from build123d import *

# Parameters (mm, degrees)
SKETCH1_W                   = 25.4
SKETCH1_H                   = 25.4
SKETCH1_W_2                 = 15.875
SKETCH1_H_2                 = 15.875
BOSS_EXTRUDE1_DEPTH         = 298
FILLET1_R                   = 1.5
F_1_4_0_25_DIAMETER_HOLE1_D = 6.35
SKETCH4_R                   = 2.2
SKETCH4_R_2                 = 2.75
CUT_EXTRUDE1_DEPTH          = 26.4


with BuildPart() as part:
    # Sketch1 → Boss-Extrude1 (new body, symmetric)
    with BuildSketch(Plane(origin=(0, 0, 0), x_dir=(1, 0, 0), z_dir=(0, 1, 0))):
        Rectangle(SKETCH1_W, SKETCH1_H)
        Rectangle(SKETCH1_W_2, SKETCH1_H_2, mode=Mode.SUBTRACT)
    extrude(amount=BOSS_EXTRUDE1_DEPTH, both=True)

    # Fillet1
    fillet1_edges = [part.edges().sort_by_distance(p)[0] for p in [
        (12.7, 0, 12.7),
        (-12.7, 0, 12.7),
        (-12.7, 0, -12.7),
        (12.7, 0, -12.7),
    ]]
    fillet(fillet1_edges, radius=FILLET1_R)

    # 1/4 (0.25) Diameter Hole1 (through all)
    with Locations(Plane(origin=(0.011805537, 289.825, -12.7), x_dir=(-1, 0, 0), z_dir=(0, 0, -1))):
        with Locations((0, 0), (0, -19), (0, -38)):
            f_1_4_0_25_diameter_hole1 = Hole(F_1_4_0_25_DIAMETER_HOLE1_D / 2)

    # Mirror1: 1/4 (0.25) Diameter Hole1 across plane
    add(f_1_4_0_25_diameter_hole1.mirror(Plane.ZX), mode=Mode.SUBTRACT)

    # Sketch4 → Cut-Extrude1 (cut, through all)
    with BuildSketch(Plane.ZY.offset(12.7)):
        with Locations((0, 134.3)):
            Circle(SKETCH4_R)
        with Locations((0, -134.3)):
            Circle(SKETCH4_R)
        with Locations((0, 238.65)):
            Circle(SKETCH4_R_2)
        with Locations((0, 226.9)):
            Circle(SKETCH4_R_2)
        with Locations((0, 215.15)):
            Circle(SKETCH4_R_2)
        with Locations((0, -215.15)):
            Circle(SKETCH4_R_2)
        with Locations((0, -226.9)):
            Circle(SKETCH4_R_2)
        with Locations((0, -238.65)):
            Circle(SKETCH4_R_2)
        with Locations((0, 190)):
            Circle(SKETCH4_R_2)
        with Locations((0, -190)):
            Circle(SKETCH4_R_2)
    extrude(amount=-CUT_EXTRUDE1_DEPTH, mode=Mode.SUBTRACT)


solid = part.part
The model under review builds one solid part; all positions refer to its coordinate system, in mm. A direction names the side the tool comes from. Coordinates: 2 decimals unless noted, no trailing zeros. Write each loop counter-clockwise with the first axis right and the second up, starting at its lowest first coordinate (ties: lowest second). Pieces come first, ordered by that corner, then holes. Notation, with made-up numbers: (-27.5, 43.25) - (10.5, 43.25) arc R28 cw to (10.5, 72.25) - close; hole circle Ø6 at (1.5, 71.5). An arc over 180 degrees is marked (long way). Answer as a JSON object with one key per item and string values. Group by question number.
1. Mouldability with a two-part tool opening along Z and no side actions: class faces 1 (the face through (-7.938, 4, 0)), 2 (the face through (8.3, 298, -0.2)), 3 (the face through (0, 4, 12.7)) as pulls with the +Z half, pulls with the -Z half, needs draft (parallel to the pull), parting line crosses it, or undercut.
2. Add section A-A (y = 119.5). Give the boundary of the cut face in (x, z).
3. To check wall thickness, follow probe 1 along Z at (x, y) = (5.5, 87.5); probe 2 along Z at (x, y) = (-9.6, -215.15). State the ranges of each line that lie inside material, in increasing order.
4. Machinability: for faces 4 (the face through (0, 4, 7.938)), 5 (the face through (8.3, -298, -0.2)), which of the approach directions +Z, -Z, +X, -X, +Y, -Y give a long, thin tool a straight path to every point of the face, cutting with its end or side? Answer none if there is none.
Findings:
{
 "1": {"face 1": "undercut", "face 2": "needs draft", "face 3": "pulls with the +Z half"},
 "2": {"outline": "(-12.7, -11.2) arc R1.5 ccw to (-11.2, -12.7) - (11.2, -12.7) arc R1.5 ccw to (12.7, -11.2) - (12.7, 11.2) arc R1.5 ccw to (11.2, 12.7) - (-11.2, 12.7) arc R1.5 ccw to (-12.7, 11.2) - close; hole (-7.94, -7.94) - (7.94, -7.94) - (7.94, 7.94) - (-7.94, 7.94) - close"},
 "3": {"probe 1": "-12.7 to -7.94, 7.94 to 12.7", "probe 2": "-12.7 to -2.75, 2.75 to 12.7"},
 "4": {"face 4": "+Y, -Y", "face 5": "+Z, -Z, +X, -X, -Y"}
}
